```python
from build123d import *

# Parameters (mm, degrees)
EXTRUDE_1_DEPTH             = 8
CUT_EXTRUDE_1_DEPTH         = 5
HOLE_WIZARD_M61_D           = 6.3
HOLE_WIZARD_M61_DEPTH       = 4.2
HOLE_WIZARD_M61_CBORE_D     = 12
HOLE_WIZARD_M61_CBORE_DEPTH = 3
FILLET_1_R                  = 1


with BuildPart() as part:
    # Эскиз1 → Бобышка-Вытянуть1 (new body, symmetric)
    with BuildSketch(Plane.XY):
        Polygon((11, 0), (-11, 0), (-11, 9.2), (-6.75, 9.2), (-6.75, 5.7), (-5.25, 4.2), (5.25, 4.2), (6.75, 5.7), (6.75, 9.2), (11, 9.2), align=None)
    extrude(amount=EXTRUDE_1_DEPTH, both=True)

    # Эскиз2 → Вырез-Вытянуть1 (cut, symmetric)
    with BuildSketch(Plane.XY):
        Polygon((-11, 7.7), (-6.75, 7.7), (-6.75, 5.7), (-5.25, 4.2), (-6.5, 4.2), (-6.5, 0), (-11, 0), align=None)
    cut_extrude_1 = extrude(amount=CUT_EXTRUDE_1_DEPTH, both=True, mode=Mode.SUBTRACT)

    # Зеркальное отражение1: Вырез-Вытянуть1 across plane
    add(cut_extrude_1.mirror(Plane(origin=(0, 0, 0), x_dir=(0, 0, 1), z_dir=(1, 0, 0))), mode=Mode.SUBTRACT)

    # Цековка для  болта с шестигранной головкой M61
    with Locations(Plane(origin=(0, 4.2, 0), x_dir=(1, 0, 0), z_dir=(0, 1, 0))):
        with Locations((0, 0)):
            CounterBoreHole(HOLE_WIZARD_M61_D / 2, HOLE_WIZARD_M61_CBORE_D / 2, HOLE_WIZARD_M61_CBORE_DEPTH, depth=HOLE_WIZARD_M61_DEPTH)

    # Скругление1
    fillet_1_edges = [part.edges().sort_by_distance(p)[0] for p in [
        (11, 4.6, 8),
        (11, 4.6, -8),
        (-11, 4.6, -8),
        (-11, 4.6, 8),
    ]]
    fillet(fillet_1_edges, radius=FILLET_1_R)


solid = part.part
```
For this review, take the finished solid that the model builds, in its own axes (mm). A direction names the side the tool comes from. Coordinates: 2 decimals unless noted, no trailing zeros. Loops run counter-clockwise (first coordinate to the right, second up) from the corner with the lowest first, then second, coordinate; pieces in that order, holes last. Notation, with made-up numbers: (67.25, -17.5) - (86.25, -17.5) arc R4 ccw to (86.25, -10.5) - close; hole circle Ø3 at (51, 19.5). An arc over 180 degrees is marked (long way). Use one line per item in the form item = value. Start each with the question number.
1) Take a section at C-C (z = 0). State the section outline as (x, y) points.
2) Take a section at A-A (y = 5). State the section outline as (x, z) points, plus the area to 3 significant figures.
3) To check wall thickness, follow probe 1 along Z at (x, y) = (7.75, 4.25); probe 2 along Z at (x, y) = (0, 0.75); probe 3 along X at (y, z) = (8.5, 4.5). State the ranges of each line that lie inside material, in increasing order. Write a range as from..to.
4) For pin 1 (4 mm diameter, centred on x = 2, y = 8, fed in from +Z); pin 2 (3 mm diameter, centred on y = 3.5, z = 1.5, fed in from +X); pin 3 (1.3 mm diameter, centred on x = 8, z = 0.5, fed in from -Y); pin 4 (5 mm diameter, centred on x = -1, z = -4.5, fed in from +Y), all flat-tipped, find the tip position at first contact; note any pin that passes through.
5) Draft analysis for pull direction X (two halves, no side actions). For faces 5 (the face through (-11, 8, 0)), 6 (the face through (-9, 4, 5)), 7 (the face through (5.99, 4.94, -6.48)), 8 (the face through (10.715, 4.536, 7.699)), state which applies: released by +X, released by -X, zero draft, split by the parting line, or undercut.
6) Take a section at D-D (y = 8.25). State the section outline as (x, z) points, plus the area to 3 significant figures.
7) For faces 1 (the face through (-6.5, 2, 0)), 2 (the face through (5.99, 4.94, 6.52)), 3 (the face through (-6, 3, 0)), 4 (the face through (9, 7.7, 0)), list the 3-axis set-ups (+Z, -Z, +X, -X, +Y, -Y) from which the entire face can be reached by the end or side of a thin tool; tool diameter is ignored.
8) Take a section at B-B (x = 0). State the section outline as (y, z) points.
From the geometry:
q1.outline = (-11, 7.7) - (-6.75, 7.7) - (-6.75, 9.2) - (-11, 9.2) - close; (-6.5, 0) - (-3.15, 0) - (-3.15, 1.2) - (-6, 1.2) - (-6, 4.2) - (-6.5, 4.2) - close; (3.15, 0) - (6.5, 0) - (6.5, 4.2) - (6, 4.2) - (6, 1.2) - (3.15, 1.2) - close; (6.75, 7.7) - (11, 7.7) - (11, 9.2) - (6.75, 9.2) - close
q2.outline = (-11, -7) arc R1 ccw to (-10, -8) - (-6.05, -8) - (-6.05, -5) - (-11, -5) - close; (-11, 5) - (-6.05, 5) - (-6.05, 8) - (-10, 8) arc R1 ccw to (-11, 7) - close; (6.05, -8) - (10, -8) arc R1 ccw to (11, -7) - (11, -5) - (6.05, -5) - close; (6.05, 5) - (11, 5) - (11, 7) arc R1 ccw to (10, 8) - (6.05, 8) - close
q2.area = 58.5 mm2
q3.probe_1 = -8..-5, 5..8
q3.probe_2 = -8..-3.15, 3.15..8
q3.probe_3 = -11..-6.75, 6.75..11
q4.pin_1 = through
q4.pin_2 = 6.5
q4.pin_3 = 7.7
q4.pin_4 = 4.2
q5.face_5 = released by -X
q5.face_6 = zero draft
q5.face_7 = undercut
q5.face_8 = released by +X
q6.outline = (-11, -7) arc R1 ccw to (-10, -8) - (-6.75, -8) - (-6.75, 8) - (-10, 8) arc R1 ccw to (-11, 7) - close; (6.75, -8) - (10, -8) arc R1 ccw to (11, -7) - (11, 7) arc R1 ccw to (10, 8) - (6.75, 8) - close
q6.area = 135 mm2
q7.face_1 = -X, +Y, -Y
q7.face_2 = +Z, -Z, +Y
q7.face_3 = +Y
q7.face_4 = +X, -X, -Y
q8.outline = (0, -8) - (4.2, -8) - (4.2, -6) - (1.2, -6) - (1.2, -3.15) - (0, -3.15) - close; (0, 3.15) - (1.2, 3.15) - (1.2, 6) - (4.2, 6) - (4.2, 8) - (0, 8) - close
